Input: dimensioned drawing with shaded views. Units: mm. Origin: part minimum x, y, z. A direction names the side the tool comes from. Coordinates: 2 decimals unless noted, no trailing zeros. Loops run counter-clockwise (first coordinate to the right, second up) from the corner with the lowest first, then second, coordinate; pieces in that order, holes last. Notation, with made-up numbers: (4, 48) - (52, 48) arc R17 cw to (52, 55) - close; hole circle Ø4 at (-23, 28.5). An arc over 180 degrees is marked (long way). Put each result on its own line as item: value. Start each with the question number.
1) Material intervals for line 1 along Y through (x, z) = (8, 36.5); line 2 along Y through (x, z) = (1.75, 8); line 3 along Z through (x, y) = (2.75, 6), sorted ascending. Write a range as from..to.
2) Section C-C on y = 37.5. Output: boundary loops of the cut face in (x, z), and give its area (3 significant figures).
3) Section B-B on y = 17.5. Output: boundary loops of the cut face in (x, z), and give its area (3 significant figures).
4) Section D-D on x = 7.5. Output: boundary loops of the cut face in (y, z) (3 decimals), and give its area (3 significant figures).
5) Draft query along Z for the marked faces 1, 2 and 3. Return one class per face: +Z half, -Z half, draft (parallel to the pull), parting line (faces both ways), or undercut.
6) Section A-A on z = 14. Output: boundary loops of the cut face in (x, y).
7) Reachability of the marked faces 4 and 5 from +Z, -Z, +X, -X, +Y, -Y: full face, straight path, thin tool, end or side. Return the list, or none.
8) Contact query for flat-ended pins moving along their axis: pin 1 Ø6.5 at (y, z) = (4, 5) entering from -X; pin 2 Ø3 at (y, z) = (35.5, 35.5) entering from -X. Output: stop coordinate, or through.
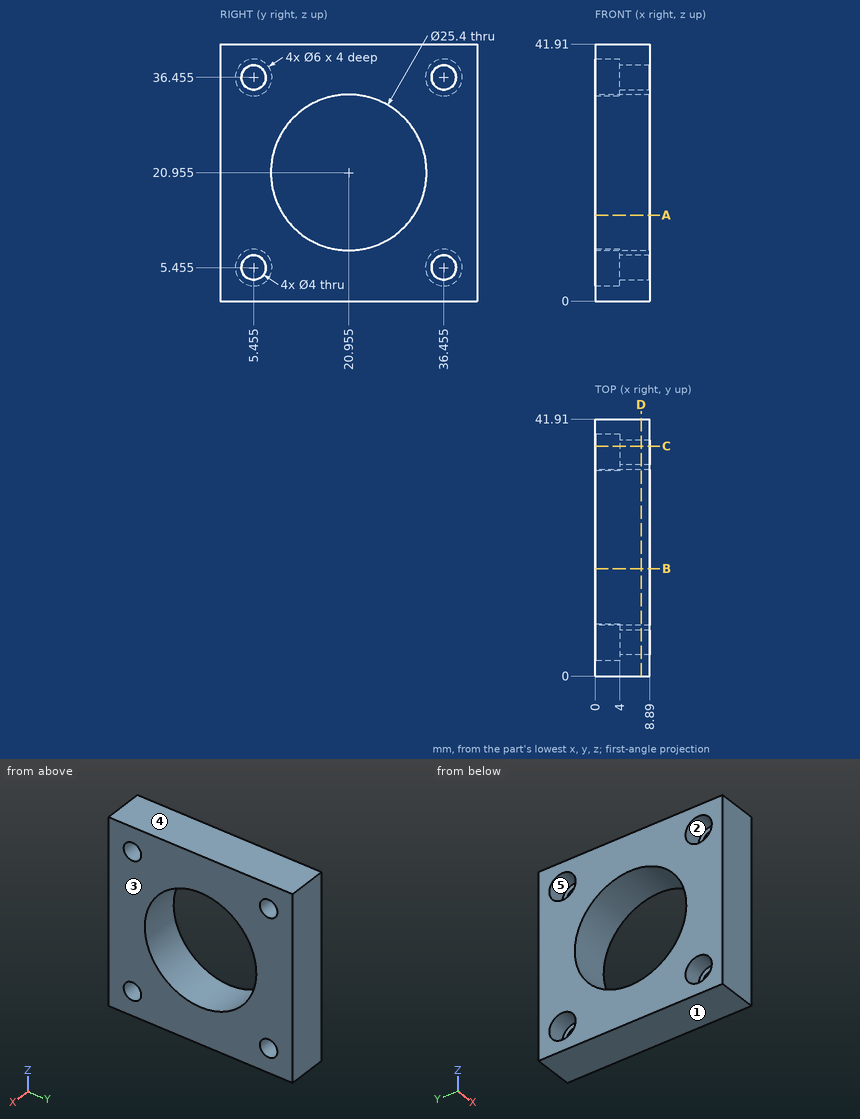
Answer block:
1. line 1: y = 0..3.46, 7.45..34.46, 38.45..41.91
1. line 2: y = 0..3.87, 7.04..34.87, 38.04..41.91
1. line 3: z = 0..2.5, 8.41..33.5, 39.41..41.91
2. outline: (0, 0) - (8.89, 0) - (8.89, 3.75) - (4, 3.75) - (4, 2.64) - (0, 2.64) - close; (0, 8.27) - (4, 8.27) - (4, 7.16) - (8.89, 7.16) - (8.89, 34.75) - (4, 34.75) - (4, 33.64) - (0, 33.64) - close; (0, 39.27) - (4, 39.27) - (4, 38.16) - (8.89, 38.16) - (8.89, 41.91) - (0, 41.91) - close
2. area: 294 mm²
3. outline: (0, 0) - (8.89, 0) - (8.89, 8.73) - (0, 8.73) - close; (0, 33.18) - (8.89, 33.18) - (8.89, 41.91) - (0, 41.91) - close
3. area: 155 mm²
4. outline: (0, 0) - (41.91, 0) - (41.91, 41.91) - (0, 41.91) - close; hole circle Ø4 at (5.455, 5.455); hole circle Ø4 at (5.455, 36.455); hole circle Ø25.4 at (20.955, 20.955); hole circle Ø4 at (36.455, 5.455); hole circle Ø4 at (36.455, 36.455)
4. area: 1,200 mm²
5. face 1: -Z half
5. face 2: undercut
5. face 3: draft
6. outline: (0, 0) - (8.89, 0) - (8.89, 10.33) - (0, 10.33) - close; (0, 31.58) - (8.89, 31.58) - (8.89, 41.91) - (0, 41.91) - close
7. face 4: +Z, +X, -X, +Y, -Y
7. face 5: -X
8. pin 1: stops at x = 0
8. pin 2: stops at x = 4
